```python
from build123d import *

# Parameters (mm, degrees)
SKETCH1_R           = 1.98968489
BOSS_EXTRUDE2_DEPTH = 22
SKETCH8_W           = 4
SKETCH8_H           = 22
BOSS_EXTRUDE4_DEPTH = 1


with BuildPart() as part:
    # Sketch1 → Boss-Extrude2 (new body)
    with BuildSketch(Plane(origin=(0, 0, 0), x_dir=(1, 0, 0), z_dir=(0, 1, 0))):
        with BuildLine():
            Line((-18.607019748, 0.497178681), (-18.607019748, 5.497178681))
            Line((-18.607019748, 5.497178681), (-14.607019748, 5.497178681))
            Line((-14.607019748, 5.497178681), (-14.607019748, -9.555359754))
            ThreePointArc((-14.607019748, -9.555359754), (-21.107019748, -14.402142963), (-27.607019748, -9.555359754))
            Line((-27.607019748, -9.555359754), (-27.607019748, 5.497178681))
            Line((-27.607019748, 5.497178681), (-23.607019748, 5.497178681))
            Line((-23.607019748, 5.497178681), (-23.607019748, 0.497178681))
            ThreePointArc((-23.607019748, 0.497178681), (-21.107019748, -2.002821319), (-18.607019748, 0.497178681))
        make_face()
        with Locations(Location((-21.107019748, -7.202821319, 0), (0, 0, 270))):
            Circle(SKETCH1_R, mode=Mode.SUBTRACT)
    extrude(amount=BOSS_EXTRUDE2_DEPTH)

    # Sketch8 → Boss-Extrude4 (add)
    with BuildSketch(Plane(origin=(0, 0, -5.497178681), x_dir=(-1, 0, 0), z_dir=(0, 0, -1))):
        with Locations((16.607019748, 11)):
            Rectangle(SKETCH8_W, SKETCH8_H)
        with Locations((25.607019748, 11)):
            Rectangle(SKETCH8_W, SKETCH8_H)
    extrude(amount=BOSS_EXTRUDE4_DEPTH)

    # Cut-Extrude1 cone 1 section (through the dimple's axis) → Cut-Extrude1 (revolve, cut)
    with BuildSketch(Plane(origin=(-14.607019748, 11, 7.202821319), x_dir=(0, 0, -1), z_dir=(0, 1, 0))):
        Polygon((0, 0), (2, 0), (0, 2), align=None)
    revolve(axis=Axis((-14.607019748, 11, 7.202821319), (-1, 0, 0)), mode=Mode.SUBTRACT)

    # Cut-Extrude1 cone 2 section (through the dimple's axis) → Cut-Extrude1 cone 2 (revolve, cut)
    with BuildSketch(Plane(origin=(-14.607019748, 16.470043573, -0.497178681), x_dir=(0, 0, -1), z_dir=(0, 1, 0))):
        Polygon((0, 0), (2, 0), (0, 2), align=None)
    revolve(axis=Axis((-14.607019748, 16.470043573, -0.497178681), (-1, 0, 0)), mode=Mode.SUBTRACT)

    # Cut-Extrude1 cone 3 section (through the dimple's axis) → Cut-Extrude1 cone 3 (revolve, cut)
    with BuildSketch(Plane(origin=(-14.607019748, 5.529956427, -0.497178681), x_dir=(0, 0, -1), z_dir=(0, 1, 0))):
        Polygon((0, 0), (2, 0), (0, 2), align=None)
    revolve(axis=Axis((-14.607019748, 5.529956427, -0.497178681), (-1, 0, 0)), mode=Mode.SUBTRACT)


solid = part.part
```
Source: CAD feature listing. Evaluate the final solid. Frame: model axes, mm. A direction names the side the tool comes from. Coordinates: 2 decimals unless noted, no trailing zeros. Loops run counter-clockwise (first coordinate to the right, second up) from the corner with the lowest first, then second, coordinate; pieces in that order, holes last. Notation, with made-up numbers: M 59,57.5 L 86,57.5 A19 ccw 86,86.5 Z; hole C 62,-37 d10. An arc over 180 degrees is marked long. Put each result on its own line as item: value. Start each with the question number.
1) Cut plane D-D on x = -18.25. Return the cut outline in (y, z).
2) Ray query, L1, parallel to X at y = 19, z = -4.5; L2, parallel to Z at x = -21, y = 16.75; L3, parallel to Z at x = -16, y = 10.5. Return the intervals inside material, ascending. Write a range as from..to.
3) Cut plane C-C on x = -20. Return the cut outline in (y, z).
4) Cut plane A-A on x = -21.5. Return the cut outline in (y, z).
5) Pull-direction query (Y, two-part tool) for faces 1 (the face through (-16.065, 5.073, -0.788)), 2 (the face through (-23.607, 11, -4)), 3 (the face through (-21, 0, 4)); classes: pulls with the +Y half, pulls with the -Y half, needs draft (parallel to the pull), parting line crosses it, or undercut.
6) Reachability of faces 4 (the face through (-21, 22, 4)), 5 (the face through (-18.607, 11, -3)) from +Z, -Z, +X, -X, +Y, -Y: full face, straight path, thin tool, end or side. Return the list, or none.
7) Contact query for a flat-ended pin moving along its axis: pin 1 Ø1.5 at (x, y) = (-21, 14.5) entering from -Z. Output: stop coordinate, or through.
8) Cut plane B-B on y = 2.25. Return the cut outline in (x, z), then the cut area to 3 significant figures.
The answers:
1. outline: M 0,-6.5 L 22,-6.5 L 22,13.77 L 0,13.77 Z
2. L1: x = -27.61..-23.61, -18.61..-14.61
2. L2: z = 2..5.22, 9.19..14.4
2. L3: z = -6.5..6.86, 7.55..12.08
3. outline: M 0,1.74 L 22,1.74 L 22,5.55 L 0,5.55 Z; M 0,8.86 L 22,8.86 L 22,14.31 L 0,14.31 Z
4. outline: M 0,1.97 L 22,1.97 L 22,5.25 L 0,5.25 Z; M 0,9.15 L 22,9.15 L 22,14.39 L 0,14.39 Z
5. face 1: undercut
5. face 2: needs draft
5. face 3: pulls with the -Y half
6. face 4: +Z, -Z, +X, -X, +Y
6. face 5: -Z, +Y, -Y
7. pin 1: stops at z = 1.85
8. outline: M -27.61,-6.5 L -23.61,-6.5 L -23.61,-0.5 A2.5 cw -18.61,-0.5 L -18.61,-6.5 L -14.61,-6.5 L -14.61,9.56 A6.78 ccw -27.61,9.56 Z; hole C -21.11,7.2 d3.98
8. area: 203 mm²
